The model under review builds one solid part; all positions refer to its coordinate system, in mm. A direction names the side the tool comes from. Give positions to 0.01 mm unless a question says otherwise; leave off trailing zeros. Loops run counter-clockwise (first coordinate to the right, second up) from the corner with the lowest first, then second, coordinate; pieces in that order, holes last. Notation, with made-up numbers: (66.5, 5) - (105.5, 5) arc R15 cw to (105.5, 20) - close; hole circle Ø6 at (-17.5, 66). An arc over 180 degrees is marked (long way). Answer as a JSON object with one key per item and string values.
from build123d import *

# Parameters (mm, degrees)
F1_DEPTH = 38.1
F2_R     = 9.525
F3_R     = 25.4
F4_R     = 16.66875
F5_DEPTH = 25.4


with BuildPart() as f1:
    # F0 (on Front) → F1 (new body, symmetric)
    with BuildSketch(Plane.XZ):
        Polygon((-41.275, 46.0375), (41.275, 46.0375), (41.275, -46.0375), (57.15, -46.0375), (57.15, 46.0375), (57.15, 61.9125), (41.275, 61.9125), (-41.275, 61.9125), (-57.15, 61.9125), (-57.15, 46.0375), (-57.15, -46.0375), (-41.275, -46.0375), align=None)
    extrude(amount=F1_DEPTH, both=True)

    # F2
    f2_edges = [f1.edges().sort_by_distance(p)[0] for p in [
        (-41.275, 0, 46.0375),
        (41.275, 0, 46.0375),
    ]]
    fillet(f2_edges, radius=F2_R)

    # F3
    f3_edges = [f1.edges().sort_by_distance(p)[0] for p in [
        (-57.15, 0, 61.9125),
        (57.15, 0, 61.9125),
    ]]
    fillet(f3_edges, radius=F3_R)

    # F4 (on face) → F5 (cut)
    with BuildSketch(Plane.XY.offset(61.9125)):
        Circle(F4_R)
    extrude(amount=-F5_DEPTH, mode=Mode.SUBTRACT)


solid = f1.part
Q1. Consider section A-A, the plane x = 0. State the section outline as (y, z) points.
Results:
{"outline": "(-38.1, 46.04) - (-16.67, 46.04) - (-16.67, 61.91) - (-38.1, 61.91) - close; (16.67, 46.04) - (38.1, 46.04) - (38.1, 61.91) - (16.67, 61.91) - close"}
Q2. Consider section C-C, the plane z = 35. State the section outline as (x, y) points (3 decimals).
Results:
{"outline": "(-57.15, -38.1) - (-41.275, -38.1) - (-41.275, 38.1) - (-57.15, 38.1) - close; (41.275, -38.1) - (57.15, -38.1) - (57.15, 38.1) - (41.275, 38.1) - close"}
Q3. For faces 5 (the face through (-49, -1, -46.038)), 6 (the face through (-15, -9, 46.038)), list the 3-axis set-ups (+Z, -Z, +X, -X, +Y, -Y) from which the entire face can be reached by the end or side of a thin tool; tool diameter is ignored.
Results:
{"face 5": "-Z, +X, -X, +Y, -Y", "face 6": "-Z, +Y, -Y"}
Q4. The part is to be moulded in two halves that separate along X. For faces 1 (the face through (41.275, -1, -4)), 2 (the face through (15.9, 5, 54.1)), 3 (the face through (-49.91, -0.53, 54.27)), 4 (the face through (-5, -38.1, 48)), say which applies: +X half, -X half, draft (parallel to the pull), parting line (faces both ways), or undercut.
Results:
{"face 1": "undercut", "face 2": "undercut", "face 3": "-X half", "face 4": "draft"}
Q5. Clearance check with flat-ended pins moving along their axes: pin 1 Ø3 at (y, z) = (-5.5, 40.5) entering from +X; pin 2 Ø6 at (x, z) = (-36.5, 4.5) entering from -Y. State where each tip first meets the part, or that it passes through.
Results:
{"pin 1": "stops at x = 57.03", "pin 2": "passes through"}
Q6. To check wall thickness, follow probe 1 along Y at (x, z) = (-1, 50); probe 2 along Y at (x, z) = (0, 50.25); probe 3 along X at (y, z) = (-11, -16) (3 decimals). State the ranges of each line that lie inside material, in increasing order. Write a range as [from, to].
Results:
{"probe 1": "y = [-38.1, -16.64], [16.64, 38.1]", "probe 2": "y = [-38.1, -16.67], [16.67, 38.1]", "probe 3": "x = [-57.15, -41.275], [41.275, 57.15]"}
